Design review of the part built by this model. Coordinates are the model's own, in mm. A direction names the side the tool comes from. Round coordinates to 2 decimals unless told otherwise and drop trailing zeros. Write each loop counter-clockwise with the first axis right and the second up, starting at its lowest first coordinate (ties: lowest second). Pieces come first, ordered by that corner, then holes. Notation, with made-up numbers: (27, 38) -> (83, 38) arc R27 cw to (83, 66) -> close; hole circle Ø10 at (67.5, 89.25). An arc over 180 degrees is marked (long way). Write item = value, one per line. Start each with the question number.
Item 1: Machinability: for faces 1 (the flat face through (-53.989, 0, 11)), 2 (the flat face through (-17.863, -1, 44)), which of the approach directions +Z, -Z, +X, -X, +Y, -Y give a long, thin tool a straight path to every point of the face, cutting with its end or side? Answer none if there is none.
Item 2: Add section B-B, the plane x = -14. State the section outline as (y, z) points.
Item 3: Add section A-A, the plane y = -1.65. State the section outline as (x, z) points, then the cut area to 3 significant figures.
Item 4: Mouldability with a two-part tool opening along Z and no side actions: class faces 3 (the flat face through (6, 0, 51.523)), 4 (the flat face through (-11, 0.508, 44)), 5 (the flat face through (-9, 2.54, 23)) as released by +Z, released by -Z, zero draft, split by the parting line, or undercut.
Item 5: Add section C-C, the plane z = 47. State the section outline as (x, y) points, then the cut area to 3 significant figures.
Item 6: Add section D-D, the plane x = -27.5. State the section outline as (y, z) points, then the cut area to 3 significant figures.
Item 7: For pin 1 Ø1 at (x, z) = (-10.5, 44.5) entering from -Y; pin 2 Ø0.6 at (y, z) = (-1.5, 44.5) entering from -X, all flat-tipped, find the tip position at first contact; note any pin that passes through.
Item 8: To check wall thickness, follow L1, parallel to X at y = -1.55, z = 42; L2, parallel to X at y = 1.35, z = 44; L3, parallel to Z at x = -47, y = -1.65. State the ranges of each line that lie inside material, in increasing order.
from build123d import *

# Parameters (mm, degrees)
F0_W          = 58.9205864817
F0_H          = 37.636497058
F0_W_2        = 32.3154758662
F1_DEPTH      = 2.54
F1_DEPTH_BACK = 2.54
F2_W          = 3.5040900111
F2_H          = 3.5040876828
F2_W_2        = 3.5040881485
F3_DEPTH      = 3.556
F4_W          = 9.6756285056
F4_H          = 1.0419934988
F5_DEPTH      = 1.524
F6_W          = 14.1413027886
F6_H          = 1.9351281226
F7_DEPTH      = 3.048


with BuildPart() as f1:
    # F0 (on Front) → F1 (new body, two sides)
    with BuildSketch(Plane.XZ) as f1_sk:
        Polygon((-25.1475647092, 51.5233650804), (-53.9889074862, 30.3038693964), (4.9316789955, 30.3038693964), align=None)
        Polygon((-25.1475647092, 51.5233650804), (4.9316789955, 30.3038693964), (37.2471548617, 30.3038693964), (37.2471548617, 51.5233650804), align=None)
        with Locations((-24.5286142454, 11.4856208675)):
            Rectangle(F0_W, F0_H)
        with Locations((21.0894169286, 11.4856208675)):
            Rectangle(F0_W_2, F0_H)
    extrude(amount=F1_DEPTH)
    extrude(f1_sk.sketch, amount=-F1_DEPTH_BACK)

    # F2 (on face) → F3 (cut)
    with BuildSketch(Plane(origin=(0, 0, -7.3326276615), x_dir=(1, 0, 0), z_dir=(0, 0, -1))):
        with Locations((-47.6945266128, 5.5805838201)):
            Rectangle(F2_W, F2_H)
        with Locations((27.3189069703, 5.5805838201)):
            Rectangle(F2_W_2, F2_H)
    extrude(amount=-F3_DEPTH, mode=Mode.SUBTRACT)

    # F4 (on face) → F5 (join)
    with BuildSketch(Plane.XZ.offset(2.54)):
        with Locations((-4.8378142528, 45.4010255635)):
            Rectangle(F4_W, F4_H)
    extrude(amount=-F5_DEPTH)

    # F6 (on face) → F7 (cut)
    with BuildSketch(Plane.XZ.offset(2.54)):
        with Locations((-10.7920466689, 44.3590339273)):
            Rectangle(F6_W, F6_H)
    extrude(amount=-F7_DEPTH, mode=Mode.SUBTRACT)


solid = f1.part
Result set:
q1.face_1 = +Z, -Z, -X, +Y, -Y
q1.face_2 = -Y
q2.outline = (-2.54, -7.33) -> (2.54, -7.33) -> (2.54, 51.52) -> (-2.54, 51.52) -> (-2.54, 45.33) -> (0.51, 45.33) -> (0.51, 43.39) -> (-2.54, 43.39) -> close
q3.outline = (-53.99, -7.33) -> (37.25, -7.33) -> (37.25, 51.52) -> (-25.15, 51.52) -> (-53.99, 30.3) -> close; hole (-17.86, 43.39) -> (-3.72, 43.39) -> (-3.72, 45.33) -> (-17.86, 45.33) -> close
q3.area = 5,040 mm²
q4.face_3 = released by +Z
q4.face_4 = undercut
q4.face_5 = zero draft
q5.outline = (-31.3, -2.54) -> (37.25, -2.54) -> (37.25, 2.54) -> (-31.3, 2.54) -> close
q5.area = 348 mm²
q6.outline = (-2.54, -7.33) -> (2.54, -7.33) -> (2.54, 49.79) -> (-2.54, 49.79) -> close
q6.area = 290 mm²
q7.pin_1 = 0.51
q7.pin_2 = -35.1
q8.L1 = -38.09 to 37.25
q8.L2 = -35.37 to 37.25
q8.L3 = -7.33 to 35.45
